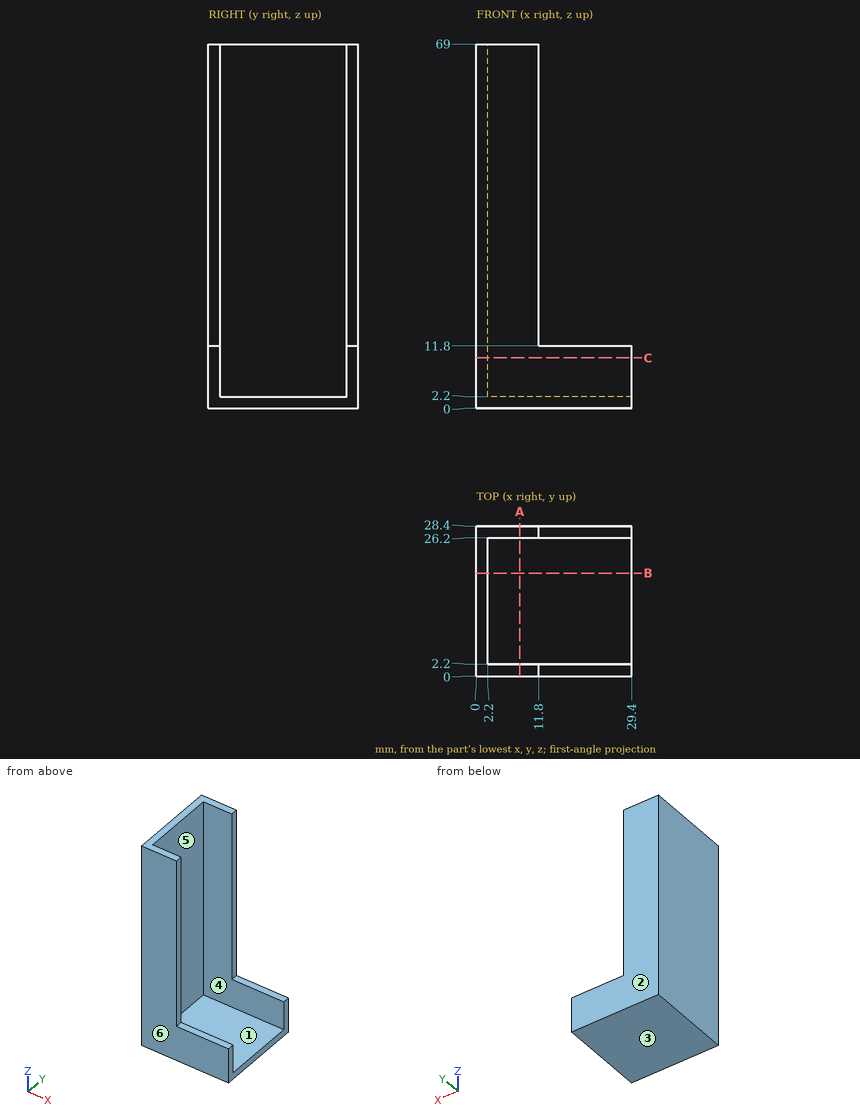
Study the drawing (mm; zero at the part's minimum x, y, z) and answer. A direction names the side the tool comes from. Round coordinates to 2 decimals unless told otherwise and drop trailing zeros. Write each loop counter-clockwise with the first axis right and the second up, starting at its lowest first coordinate (ties: lowest second). Pieces come first, ordered by that corner, then holes.
Q1. The mould has two halves that part along Y. Classify the marked faces 1, 2, 3 and 4: released by +Y, released by -Y, zero draft, split by the parting line, or undercut.
Values:
face 1: undercut
face 2: released by +Y
face 3: zero draft
face 4: undercut
Q2. Flat-ended cylindrical pins translate along their axes: P1, Ø5, axis at x = 15, z = 15.5, coming from the -Y side; P2, Ø1.8, axis at x = 21.5, y = 27.5, coming from the +Z side; P3, Ø1, axis at y = 17, z = 53, coming from the +X side; P4, Ø0.7, axis at y = 0.5, z = 32, coming from the +X side. Find the tip coordinate at first contact, or state that the pin passes through.
Values:
P1: passes through
P2: stops at z = 11.8
P3: stops at x = 2.2
P4: stops at x = 11.8
Q3. Find section A-A on x = 8.25. Determine the outline of the cut face in (y, z).
Values:
outline: (0, 0) - (28.4, 0) - (28.4, 69) - (26.2, 69) - (26.2, 2.2) - (2.2, 2.2) - (2.2, 69) - (0, 69) - close
Q4. Find section C-C on z = 9.5. Determine the outline of the cut face in (x, y), and give its area (3 significant figures).
Values:
outline: (0, 0) - (29.4, 0) - (29.4, 2.2) - (2.2, 2.2) - (2.2, 26.2) - (29.4, 26.2) - (29.4, 28.4) - (0, 28.4) - close
area: 182 mm2
Q5. A tool of negligible diameter and unlimited length cuts with its end or side. For the marked faces 5 and 6, from which of +Z, -Z, +X, -X, +Y, -Y can it reach the whole face along a straight path? Write none if from no direction.
Values:
face 5: +Z, +X
face 6: +Z, -Z, +X, -X, -Y
Q6. Find section B-B on y = 19.5. Determine the outline of the cut face in (x, z).
Values:
outline: (0, 0) - (29.4, 0) - (29.4, 2.2) - (2.2, 2.2) - (2.2, 69) - (0, 69) - close
Q7. Straight lines are drawn through the part: line 1 (Y direction, x = 11, z = 41); line 2 (X direction, y = 26.25, z = 66); line 3 (Z direction, x = 18.75, y = 8.75). For each, find the intervals that lie inside material, in ascending order.
Values:
line 1: y = 0 to 2.2, 26.2 to 28.4
line 2: x = 0 to 11.8
line 3: z = 0 to 2.2
